Verification items for this drawing (mm, ordinates from the low corner). Round coordinates to 2 decimals unless told otherwise and drop trailing zeros. Write each loop counter-clockwise with the first axis right and the second up, starting at its lowest first coordinate (ties: lowest second). Pieces come first, ordered by that corner, then holes.
Item 1: Cross-section at B-B (x = 2). Enter the section's corners in (y, z).
Item 2: Cross-section at C-C (y = 12.25). Enter the section's corners in (x, z).
Item 3: Depth check by flat-ended pin: P1, Ø2.5, axis at x = 3.25, y = 12.5, coming from the +Z side. Enter the tip coordinate at first touch or a pass-through.
Item 4: Draft check along X on the marked faces 1, 2, 3 and 4. Enter one of: pulls with the +X half, pulls with the -X half, needs draft (parallel to the pull), parting line crosses it, or undercut.
Item 5: Cross-section at D-D (y = 14.5). Enter the section's corners in (x, z).
Item 6: Scan lines: probe 1 along Y at (x, z) = (3.25, 0.2); probe 2 along X at (y, z) = (12.5, 0.5); probe 3 along Y at (x, z) = (4, 0.75). Record each from-to range of solid material in increasing order.
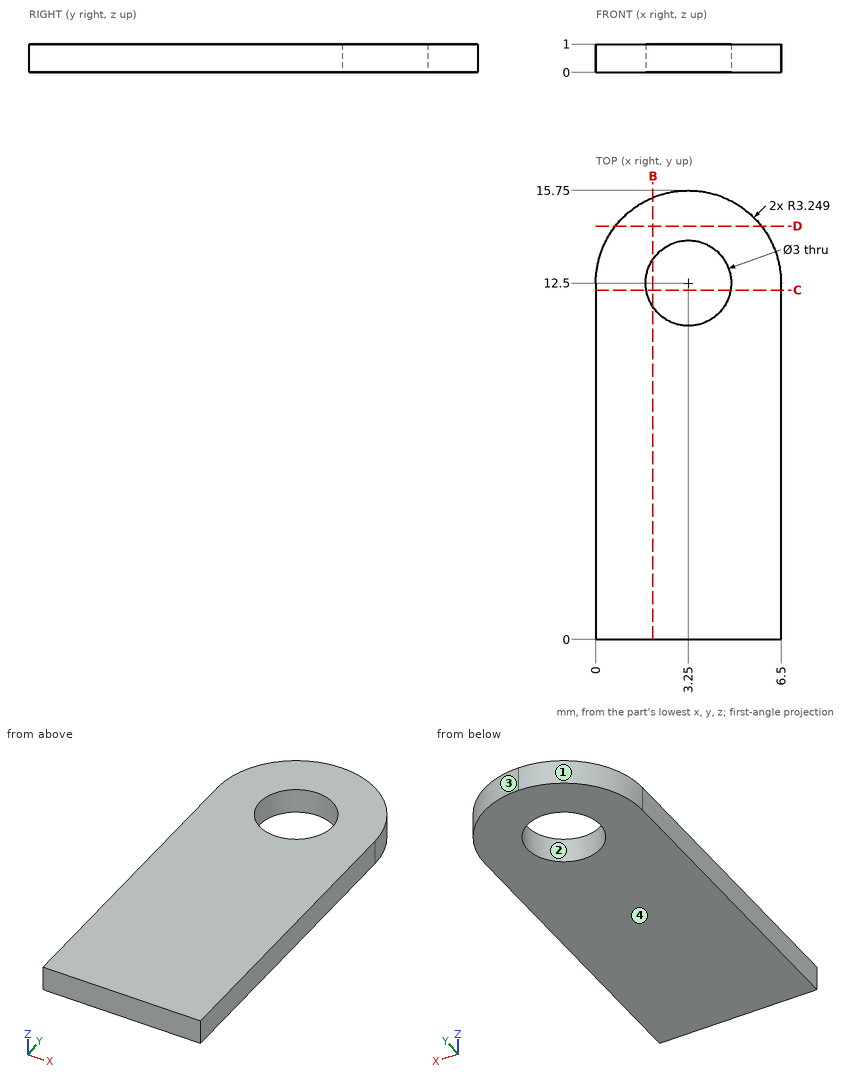
Resolved:
1. outline: (0, 0) - (11.67, 0) - (11.67, 1) - (0, 1) - close; (13.33, 0) - (15.5, 0) - (15.5, 1) - (13.33, 1) - close
2. outline: (0, 0) - (1.77, 0) - (1.77, 1) - (0, 1) - close; (4.73, 0) - (6.5, 0) - (6.5, 1) - (4.73, 1) - close
3. P1: passes through
4. face 1: pulls with the -X half
4. face 2: undercut
4. face 3: pulls with the +X half
4. face 4: needs draft
5. outline: (0.69, 0) - (5.81, 0) - (5.81, 1) - (0.69, 1) - close
6. probe 1: y = 0 to 11, 14 to 15.75
6. probe 2: x = 0 to 1.75, 4.75 to 6.5
6. probe 3: y = 0 to 11.2, 13.8 to 15.66
